Can you work these out from the model? Positions are in its coordinate system, mm. Face numbers are marked on the shaded views. Give positions to 0.01 mm unless a question says otherwise; leave off trailing zeros. Write each loop counter-clockwise with the first axis right and the second up, starting at its lowest first coordinate (ties: lowest second). Pieces come first, ordered by that corner, then holes. Notation, with made-up numbers: (70.25, -18) - (110.25, -18) arc R18 ccw to (110.25, -7) - close; hole circle Ø7 at (76.25, -29.5). An arc over 180 degrees is marked (long way). Use a Markdown table: item, result. Add a question column.
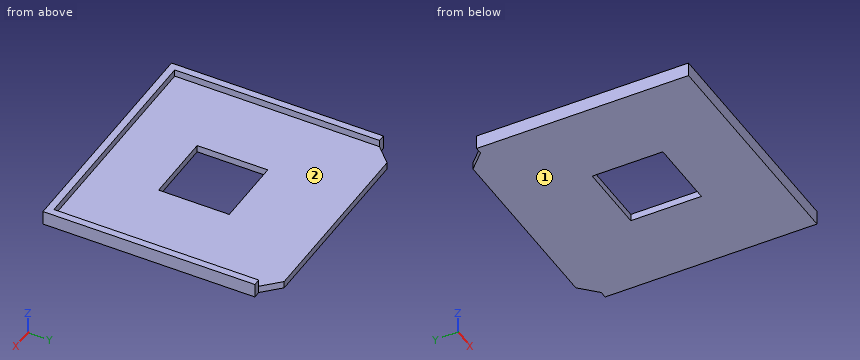
```python
from build123d import *

# Parameters (mm, degrees)
SALIENTE_EXTRUIR1_DEPTH = 3
CROQUIS3_W              = 30
CROQUIS3_H              = 30
CORTAR_EXTRUIR1_DEPTH   = 3
SALIENTE_EXTRUIR2_DEPTH = 3


with BuildPart() as part:
    # Croquis1 → Saliente-Extruir1 (new body)
    with BuildSketch(Plane.XY):
        Polygon((-50, 45), (-47, 45), (-40, 52), (40, 52), (47, 45), (50, 45), (50, -45), (-50, -45), align=None)
    extrude(amount=SALIENTE_EXTRUIR1_DEPTH)

    # Croquis3 → Cortar-Extruir1 (cut)
    with BuildSketch(Plane.XY.offset(3)):
        Rectangle(CROQUIS3_W, CROQUIS3_H)
    extrude(amount=-CORTAR_EXTRUIR1_DEPTH, mode=Mode.SUBTRACT)

    # Croquis4 → Saliente-Extruir2 (add)
    with BuildSketch(Plane.XY.offset(3)):
        Polygon((-50, 45), (-47, 45), (-47, -42), (47, -42), (47, 45), (50, 45), (50, -45), (-50, -45), align=None)
    extrude(amount=SALIENTE_EXTRUIR2_DEPTH)


solid = part.part
```
Q1. If we mould it in two halves opening along X, with no side actions, what happens to the marked faces 1 and 2? For each: released by +X, released by -X, zero draft, split by the parting line, or undercut.
Q2. Suppose I cut it at B-B (z = 4.35). Please give me the cut outline in (x, y).
Q3. Suppose I cut it at A-A (x = -6). Please give me the cut outline in (y, z), and give its area (3 significant figures).
Q4. If I drill on probe 1 along X at (y, z) = (-19, 3.9); probe 2 along X at (y, z) = (14.5, 1.65); probe 3 along Z at (x, y) = (40, 48.5), over which ranges is the centre line in solid material (lowest first)? Write a range as [from, to].
Q5. I'm going to push flat-ended pins straight in: P1, Ø4, axis at x = -29, y = -33, coming from the +Z side; P2, Ø0.9, axis at x = 49, z = 4, coming from the +Y side; P3, Ø2, axis at x = 31, z = 5.5, coming from the +Y side. Where does each tip first touch, or does it pass through?
Q6. Suppose I cut it at C-C (y = 18.5). Please give me the cut outline in (x, z), and give its area (3 significant figures).
Q7. Suppose I cut it at D-D (x = -19). Please give me the cut outline in (y, z).
Derived:
| question | item | result |
|---|---|---|
| 1 | face 1 | zero draft |
| 1 | face 2 | undercut |
| 2 | outline | (-50, -45) - (50, -45) - (50, 45) - (47, 45) - (47, -42) - (-47, -42) - (-47, 45) - (-50, 45) - close |
| 3 | outline | (-45, 0) - (-15, 0) - (-15, 3) - (-42, 3) - (-42, 6) - (-45, 6) - close; (15, 0) - (52, 0) - (52, 3) - (15, 3) - close |
| 3 | area | 210 mm² |
| 4 | probe 1 | [-50, -47], [47, 50] |
| 4 | probe 2 | [-50, -15], [15, 50] |
| 4 | probe 3 | [0, 3] |
| 5 | P1 | z = 3 |
| 5 | P2 | y = 45 |
| 5 | P3 | y = -42 |
| 6 | outline | (-50, 0) - (50, 0) - (50, 6) - (47, 6) - (47, 3) - (-47, 3) - (-47, 6) - (-50, 6) - close |
| 6 | area | 318 mm² |
| 7 | outline | (-45, 0) - (52, 0) - (52, 3) - (-42, 3) - (-42, 6) - (-45, 6) - close |
